Input: part model. Units: mm. Frame: model coordinates. A direction names the side the tool comes from. Round coordinates to 2 decimals unless told otherwise and drop trailing zeros. Loops run counter-clockwise (first coordinate to the right, second up) from the corner with the lowest first, then second, coordinate; pieces in that order, holes last. Notation, with made-up numbers: (-26, 89) -> (32, 89) arc R16 cw to (32, 105) -> close; hole circle Ø3 at (47, 4.25). An arc over 180 degrees is marked (long way). Answer as a JSON object with one key per item and string values. Group by question number.
Item 1: Set-up query: faces 4 (the flat face through (0, 2.1, -2)), 5 (the flat face through (-2.291, 4, 2)), 6 (the flat face through (0, 2, 0)), 7 (the flat face through (2.291, 4, 2)), 8 (the flat face through (0, 2.1, 2.7)). Return all of +Z, -Z, +X, -X, +Y, -Y with unobstructed straight access to the full face (end or side cutting, diameter ignored); none if empty.
Item 2: Pin query (flat end, axial travel): pin 1 (1.2 mm diameter, centred on x = 0, z = 0, fed in from -Y); pin 2 (1.6 mm diameter, centred on y = 4.5, z = 2.5, fed in from -X); pin 3 (1 mm diameter, centred on y = 6, z = -0.5, fed in from +X). Return the tip coordinate at first contact, or that it passes through.
Item 3: Section query B-B on y = 4.75. Return loops of the section in (x, z), and give its area (3 significant figures).
Item 4: Section query D-D on y = 1.75. Return loops of the section in (x, z), and give its area (3 significant figures).
Item 5: Section query A-A on x = 0. Return loops of the section in (y, z).
Item 6: Draft query along X for faces 1 (the cylindrical face through (0.17, 1.489, -2.494)), 2 (the cylindrical face through (-1, 1, 0)), 3 (the flat face through (0, 5, -1)). Return one class per face: released by +X, released by -X, zero draft, split by the parting line, or undercut.
Item 7: Section query C-C on z = 0. Return loops of the section in (x, y).
Item 8: Material intervals for line 1 (X direction, y = 1.5, z = 0); line 2 (Y direction, x = -0.4, z = -1.35); line 3 (X direction, y = 2.5, z = 1.05), sorted ascending. Write a range as [from, to].
from build123d import *

# Parameters (mm, degrees)
SKETCH1_R           = 2.5
SKETCH1_R_2         = 1
BOSS_EXTRUDE2_DEPTH = 2.1
BOSS_EXTRUDE3_DEPTH = 1
SKETCH4_R           = 1
CUT_EXTRUDE13_DEPTH = 2
SKETCH6_OUTSIDE_W   = 8.99
SKETCH6_OUTSIDE_H   = 8.99
SKETCH6_OUTSIDE_R   = 2.5
CUT_EXTRUDE14_DEPTH = 8.842193571
BOSS_EXTRUDE4_START = 2
BOSS_EXTRUDE4_DEPTH = 2


with BuildPart() as part:
    # Sketch1 → Boss-Extrude2 (new body)
    with BuildSketch(Plane(origin=(0, 0, 0), x_dir=(1, 0, 0), z_dir=(0, 1, 0))):
        with Locations(Location((0, 0, 0), (0, 0, 270))):
            Circle(SKETCH1_R)
        with Locations(Location((0, 0, 0), (0, 0, 270))):
            Circle(SKETCH1_R_2, mode=Mode.SUBTRACT)
    extrude(amount=BOSS_EXTRUDE2_DEPTH)

    # Sketch2 → Boss-Extrude3 (add, symmetric)
    with BuildSketch(Plane.XY):
        with BuildLine():
            Line((2.5, 4.5), (2.5, 0))
            Line((2.5, 0), (-2.5, 0))
            Line((-2.5, 0), (-2.5, 4.5))
            ThreePointArc((-2.5, 4.5), (0, 7), (2.5, 4.5))
        make_face()
    extrude(amount=BOSS_EXTRUDE3_DEPTH, both=True)

    # Sketch4 → Cut-Extrude13 (cut)
    with BuildSketch(Plane.XZ):
        with Locations(Location((0, 0, 0), (0, 0, 270))):
            Circle(SKETCH4_R)
    extrude(amount=-CUT_EXTRUDE13_DEPTH, mode=Mode.SUBTRACT)

    # Sketch6 outside → Cut-Extrude14 (cut, through all)
    with BuildSketch(Plane.XZ):
        Rectangle(SKETCH6_OUTSIDE_W, SKETCH6_OUTSIDE_H)
        with Locations(Location((0, 0, 0), (0, 0, 336.421821522))):
            Circle(SKETCH6_OUTSIDE_R, mode=Mode.SUBTRACT)
    extrude(amount=-CUT_EXTRUDE14_DEPTH, mode=Mode.SUBTRACT)

    # Sketch7 → Boss-Extrude4 (add)
    with BuildSketch(Plane.XY.offset(1).offset(BOSS_EXTRUDE4_START)):
        with BuildLine():
            Line((2.291287847, 2.1), (2.291287847, 5.5))
            ThreePointArc((2.291287847, 5.5), (0, 7), (-2.291287847, 5.5))
            Line((-2.291287847, 5.5), (-2.291287847, 2.1))
            Line((-2.291287847, 2.1), (2.291287847, 2.1))
        make_face()
    extrude(amount=-BOSS_EXTRUDE4_DEPTH)

    # Sketch9 → Cut-Revolve1 (revolve, cut)
    with BuildSketch(Plane.XY.offset(3)):
        with BuildLine():
            Line((-1.5, 4.5), (1.5, 4.5))
            ThreePointArc((1.5, 4.5), (0, 6), (-1.5, 4.5))
        make_face()
    revolve(axis=Axis((-1.5, 4.5, 3), (1, 0, 0)), mode=Mode.SUBTRACT)


solid = part.part
Solved:
{
 "1": {"face 4": "-Z, +X, -X, +Y", "face 5": "+Z, -X, +Y, -Y", "face 6": "-Y", "face 7": "+Z, +X, +Y, -Y", "face 8": "+Z, -Y"},
 "2": {"pin 1": "y = 2", "pin 2": "x = -2.29", "pin 3": "x = 2.29"},
 "3": {"outline": "(-2.49, -0.25) arc R2.5 ccw to (-2.29, -1) -> (2.29, -1) arc R2.5 ccw to (2.49, -0.25) -> (2.49, 0.25) arc R2.5 ccw to (2.29, 1) -> (2.29, 3) -> (1.48, 3) arc R1.48 cw to (-1.48, 3) -> (-2.29, 3) -> (-2.29, 1) arc R2.5 ccw to (-2.49, 0.25) -> close", "area": "15.4 mm²"},
 "4": {"outline": "circle Ø5 at (0, 0); hole circle Ø2 at (0, 0)", "area": "16.5 mm²"},
 "5": {"outline": "(0, -2.5) -> (2.1, -2.5) -> (2.1, -1) -> (7, -1) -> (7, 3) -> (6, 3) arc R1.5 cw to (3, 3) -> (2.1, 3) -> (2.1, 2.5) -> (0, 2.5) -> (0, 1) -> (2, 1) -> (2, -1) -> (0, -1) -> close"},
 "6": {"face 1": "split by the parting line", "face 2": "undercut", "face 3": "zero draft"},
 "7": {"outline": "(-2.5, 0) -> (-1, 0) -> (-1, 2) -> (1, 2) -> (1, 0) -> (2.5, 0) -> (2.5, 4.5) arc R2.5 ccw to (-2.5, 4.5) -> close"},
 "8": {"line 1": "[-2.5, -1], [1, 2.5]", "line 2": "[0, 2.1]", "line 3": "[-2.29, 2.29]"}
}
